Here's how the part is built. I have some questions about the finished solid (model axes, mm). Face numbers are marked on the shaded views. A direction names the side the tool comes from. Round coordinates to 2 decimals unless told otherwise and drop trailing zeros. Loops run counter-clockwise (first coordinate to the right, second up) from the corner with the lowest first, then second, coordinate; pieces in that order, holes last. Notation, with made-up numbers: M 16.25,7.25 L 40.25,7.25 A37 cw 40.25,43.25 Z; hole C 3,-37.5 d10. An arc over 180 degrees is marked long. Answer as a JSON object with one key per item and string values.
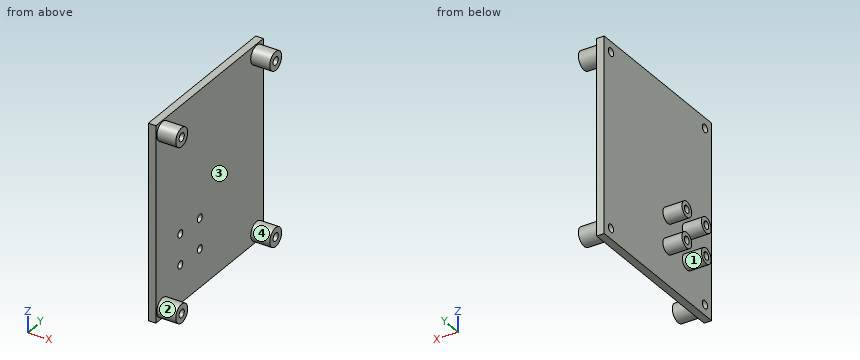
from build123d import *

# Parameters (mm, degrees)
SKETCH1_W           = 65
SKETCH1_H           = 56
BOSS_EXTRUDE1_DEPTH = 2.54
SKETCH2_R           = 3.1
SKETCH2_R_2         = 1.349999967
SKETCH2_R_3         = 1.35
BOSS_EXTRUDE2_DEPTH = 6.35
SKETCH3_R           = 2.54
SKETCH3_R_2         = 1.27
BOSS_EXTRUDE3_DEPTH = 6.35
SKETCH4_R           = 1.349999967
SKETCH4_R_2         = 1.35
SKETCH4_R_3         = 1.27
CUT_EXTRUDE1_DEPTH  = 12.7


with BuildPart() as part:
    # Sketch1 → Boss-Extrude1 (new body)
    with BuildSketch(Plane(origin=(0, 0, 0), x_dir=(0, 0, -1), z_dir=(1, 0, 0))):
        with Locations((-303.603151862, 66.376790831)):
            Rectangle(SKETCH1_W, SKETCH1_H)
    extrude(amount=BOSS_EXTRUDE1_DEPTH)

    # Sketch2 → Boss-Extrude2 (add)
    with BuildSketch(Plane(origin=(2.54, 0, 0), x_dir=(0, 0, -1), z_dir=(1, 0, 0))):
        with Locations((-332.603151862, 90.876790831)):
            Circle(SKETCH2_R)
        with Locations((-332.603151862, 90.876790831)):
            Circle(SKETCH2_R_2, mode=Mode.SUBTRACT)
        with Locations((-274.603151862, 90.876790831)):
            Circle(SKETCH2_R)
        with Locations((-274.603151862, 90.876790831)):
            Circle(SKETCH2_R_3, mode=Mode.SUBTRACT)
        with Locations((-274.603151862, 41.876790831)):
            Circle(SKETCH2_R)
        with Locations((-274.603151862, 41.876790831)):
            Circle(SKETCH2_R_3, mode=Mode.SUBTRACT)
        with Locations((-332.603151862, 41.876790831)):
            Circle(SKETCH2_R)
        with Locations((-332.603151862, 41.876790831)):
            Circle(SKETCH2_R_3, mode=Mode.SUBTRACT)
    extrude(amount=BOSS_EXTRUDE2_DEPTH)

    # Sketch3 → Boss-Extrude3 (add)
    with BuildSketch(Plane.ZY):
        with Locations((283.803151862, 61.236790831)):
            Circle(SKETCH3_R)
        with Locations((283.803151862, 61.236790831)):
            Circle(SKETCH3_R_2, mode=Mode.SUBTRACT)
        with Locations((293.963151862, 61.236790831)):
            Circle(SKETCH3_R)
        with Locations((293.963151862, 61.236790831)):
            Circle(SKETCH3_R_2, mode=Mode.SUBTRACT)
        with Locations((283.803151862, 51.076790831)):
            Circle(SKETCH3_R)
        with Locations((283.803151862, 51.076790831)):
            Circle(SKETCH3_R_2, mode=Mode.SUBTRACT)
        with Locations((293.963151862, 51.076790831)):
            Circle(SKETCH3_R)
        with Locations((293.963151862, 51.076790831)):
            Circle(SKETCH3_R_2, mode=Mode.SUBTRACT)
    extrude(amount=BOSS_EXTRUDE3_DEPTH)

    # Sketch4 → Cut-Extrude1 (cut, symmetric)
    with BuildSketch(Plane(origin=(2.54, 0, 0), x_dir=(0, 0, -1), z_dir=(1, 0, 0))):
        with Locations((-332.603151862, 90.876790831)):
            Circle(SKETCH4_R)
        with Locations((-274.603151862, 90.876790831)):
            Circle(SKETCH4_R_2)
        with Locations((-274.603151862, 41.876790831)):
            Circle(SKETCH4_R_2)
        with Locations((-332.603151862, 41.876790831)):
            Circle(SKETCH4_R_2)
        with Locations((-283.803151862, 61.236790831)):
            Circle(SKETCH4_R_3)
        with Locations((-293.963151862, 61.236790831)):
            Circle(SKETCH4_R_3)
        with Locations((-283.803151862, 51.076790831)):
            Circle(SKETCH4_R_3)
        with Locations((-293.963151862, 51.076790831)):
            Circle(SKETCH4_R_3)
    extrude(amount=CUT_EXTRUDE1_DEPTH, both=True, mode=Mode.SUBTRACT)


solid = part.part
Item 1: I want a section at D-D, the plane z = 326.5. Please give me the cut outline in (x, y).
Resolved:
{"outline": "M 0,38.38 L 2.54,38.38 L 2.54,94.38 L 0,94.38 Z"}
Item 2: I'm going to push a flat-ended pin straight in: pin 1 Ø10 at (y, z) = (67.5, 313.5) entering from +X. Where does the tip first touch, or does it pass through?
Resolved:
{"pin 1": "x = 2.54"}
Item 3: I want a section at B-B, the plane x = 4.5. Please give me the cut outline in (y, z), then the cut area to 3 significant figures.
Resolved:
{"outline": "C 41.88,274.6 d6.2; C 41.88,332.6 d6.2; C 90.88,274.6 d6.2; C 90.88,332.6 d6.2; hole C 41.88,274.6 d2.7; hole C 41.88,332.6 d2.7; hole C 90.88,274.6 d2.7; hole C 90.88,332.6 d2.7", "area": "97.9 mm²"}
Item 4: If we mould it in two halves opening along Z, with no side actions, what happens to the marked faces 3 and 4? For each: pulls with the +Z half, pulls with the -Z half, needs draft (parallel to the pull), parting line crosses it, or undercut.
Resolved:
{"face 3": "undercut", "face 4": "undercut"}
Item 5: On a 3-axis mill with a long thin cutter (end or side, diameter ignored), from which of +Z, -Z, +X, -X, +Y, -Y can I reach the whole of each face in a straight line? I mean the marked faces 1 and 2. Say none if no direction works.
Resolved:
{"face 1": "-X", "face 2": "+X"}
Item 6: I want a section at C-C, the plane y = 76.5. Please give me the cut outline in (x, z), then the cut area to 3 significant figures.
Resolved:
{"outline": "M 0,271.1 L 2.54,271.1 L 2.54,336.1 L 0,336.1 Z", "area": "165 mm²"}
Item 7: I want a section at A-A, the plane x = -3. Please give me the cut outline in (y, z).
Resolved:
{"outline": "C 51.08,283.8 d5.08; C 51.08,293.96 d5.08; C 61.24,283.8 d5.08; C 61.24,293.96 d5.08; hole C 51.08,283.8 d2.54; hole C 51.08,293.96 d2.54; hole C 61.24,283.8 d2.54; hole C 61.24,293.96 d2.54"}
Item 8: Please list where these lines run through material, in increasing order: probe 1 along Z at (x, y) = (-1.75, 52); probe 2 along X at (y, z) = (79, 303.5); probe 3 along X at (y, z) = (52.5, 284). Write a range as from..to.
Resolved:
{"probe 1": "281.44..282.93, 284.68..286.17, 291.6..293.09, 294.84..296.33", "probe 2": "0..2.54", "probe 3": "-6.35..2.54"}
